For this review, take the finished solid that the model builds, in its own axes (mm). Face numbers are marked on the shaded views. A direction names the side the tool comes from. Coordinates: 2 decimals unless noted, no trailing zeros. Write each loop counter-clockwise with the first axis right and the second up, starting at its lowest first coordinate (ties: lowest second). Pieces come first, ordered by that corner, then holes. Notation, with made-up numbers: (83.25, 45.25) -> (102.25, 45.25) arc R4 cw to (102.25, 52.25) -> close; hole circle Ø7 at (35, 23). An arc over 180 degrees is marked (long way). Put each result on its own line as item: value. Start each with the question number.
Item 1: Insertion check: P1, Ø5.5, axis at x = 1, z = -11, coming from the +Y side; P2, Ø5, axis at x = -5, z = 13, coming from the -Y side; P3, Ø8, axis at x = 13, y = 57.5, coming from the -Z side. Each pin has a flat end and moves straight along its axis. Give the tip position at first contact, or say it passes through.
Item 2: Consider section D-D on y = 58.5. Give the boundary of the cut face in (x, z), and give its area (3 significant figures).
Item 3: Consider section B-B on y = 14. Give the boundary of the cut face in (x, z).
Item 4: To check wall thickness, follow L1, parallel to Y at x = -2, z = -10.5; L2, parallel to Z at x = 6, y = 49.5; L3, parallel to Y at x = 4.5, z = 17. State the ranges of each line that lie inside material, in increasing order.
Item 5: For the marked faces 1, 2 and 3, list the 3-axis set-ups (+Z, -Z, +X, -X, +Y, -Y) from which the entire face can be reached by the end or side of a thin tool; tool diameter is ignored.
Item 6: Consider section C-C on z = 4.5. Give the boundary of the cut face in (x, y), and give its area (3 significant figures).
Item 7: Consider section A-A on x = 0. Give the boundary of the cut face in (y, z), and give its area (3 significant figures).
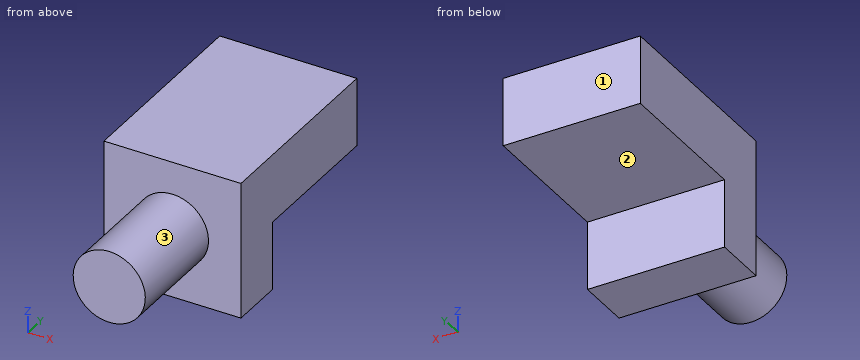
```python
from build123d import *

# Parameters (mm, degrees)
SKETCH1_R           = 10
BOSS_EXTRUDE1_DEPTH = 30
SKETCH2_W           = 38
SKETCH2_H           = 38
BOSS_EXTRUDE2_DEPTH = 15
SKETCH3_W           = 38
SKETCH3_H           = 19
BOSS_EXTRUDE3_DEPTH = 40


with BuildPart() as part:
    # Sketch1 → Boss-Extrude1 (new body)
    with BuildSketch(Plane(origin=(0, 0, 0), x_dir=(1, 0, 0), z_dir=(0, 1, 0))):
        with Locations(Location((0, 0, 0), (0, 0, 270))):
            Circle(SKETCH1_R)
    extrude(amount=BOSS_EXTRUDE1_DEPTH)

    # Sketch2 → Boss-Extrude2 (add)
    with BuildSketch(Plane(origin=(0, 30, 0), x_dir=(1, 0, 0), z_dir=(0, 1, 0))):
        Rectangle(SKETCH2_W, SKETCH2_H)
    extrude(amount=BOSS_EXTRUDE2_DEPTH)

    # Sketch3 → Boss-Extrude3 (add)
    with BuildSketch(Plane(origin=(0, 45, 0), x_dir=(1, 0, 0), z_dir=(0, 1, 0))):
        with Locations((0, -9.5)):
            Rectangle(SKETCH3_W, SKETCH3_H)
    extrude(amount=BOSS_EXTRUDE3_DEPTH)


solid = part.part
```
Return value:
1. P1: y = 45
1. P2: y = 30
1. P3: z = 0
2. outline: (-19, 0) -> (19, 0) -> (19, 19) -> (-19, 19) -> close
2. area: 722 mm^2
3. outline: circle Ø20 at (0, 0)
4. L1: 30 to 45
4. L2: 0 to 19
4. L3: 30 to 85
5. face 1: +Z, -Z, +X, -X, +Y
5. face 2: -Z, +X, -X, +Y
5. face 3: -Y
6. outline: (-19, 30) -> (-8.93, 30) -> (-8.93, 0) -> (8.93, 0) -> (8.93, 30) -> (19, 30) -> (19, 85) -> (-19, 85) -> close
6. area: 2,630 mm^2
7. outline: (0, -10) -> (30, -10) -> (30, -19) -> (45, -19) -> (45, 0) -> (85, 0) -> (85, 19) -> (30, 19) -> (30, 10) -> (0, 10) -> close
7. area: 1,930 mm^2
